Part model, mm, in its own coordinate system. Face numbers are marked on the shaded views. Round coordinates to 2 decimals unless told otherwise and drop trailing zeros. Order: outer loops, then holes, each group sorted by start corner. A loop starts at its lowest first (then second) coordinate and runs counter-clockwise, first axis right, second up. Notation, with made-up numbers: (87.5, 77) - (141.5, 77) arc R17 ccw to (141.5, 96) - close; hole circle Ø2 at (25.25, -23). An arc over 180 degrees is marked (long way). Return JSON: item names as keys, results as strings. Group by question number.
Item 1: Saw through at B-B on z = 1.35. List the corners of the cut face in (x, y).
Item 2: Saw through at C-C on y = 0.5. List the corners of the cut face in (x, z) (3 decimals), and give its area (3 significant figures).
Item 3: Probe probe 1 along Y at (x, z) = (0, 0.95); probe 2 along Z at (x, y) = (-3.75, -1); probe 3 along Z at (x, y) = (0.75, -3.75). List the from-to ranges inside material, lowest first.
Item 4: Two-plate mould, pull along Y, no slides. Class the marked faces 1, 2 and 3: released by +Y, released by -Y, zero draft, split by the parting line, or undercut.
Item 5: Saw through at A-A on x = 0. List the corners of the cut face in (y, z).
Item 6: Saw through at D-D on x = 5.25. List the corners of the cut face in (y, z), and give its area (3 significant figures).
Item 7: Drop a flat-ended pin along its axis: pin 1 (1 mm diameter, centred on y = -3, z = 1.5, fed in from -X). Give the stop position or say it passes through.
```python
from build123d import *

# Parameters (mm, degrees)
F0_R          = 2.3
F1_DEPTH      = 3
F2_R          = 72.2
F3_DEPTH      = 25
F3_DEPTH_BACK = 25


with BuildPart() as f1:
    # F0 (on Top) → F1 (new body)
    with BuildSketch(Plane.XY):
        with BuildLine():
            Line((-6.5268066341, 0), (-3.8303570799, -3.2137773166))
            ThreePointArc((-3.8303570799, -3.2137773166), (0, -5), (3.8303570799, -3.2137773166))
            Line((3.8303570799, -3.2137773166), (6.5268066341, 0))
            Line((6.5268066341, 0), (3.8303570799, 3.2137773166))
            ThreePointArc((3.8303570799, 3.2137773166), (0, 5), (-3.8303570799, 3.2137773166))
            Line((-3.8303570799, 3.2137773166), (-6.5268066341, 0))
        make_face()
        Circle(F0_R, mode=Mode.SUBTRACT)
    extrude(amount=F1_DEPTH)

    # F2 (on Front) → F3 (cut, two sides)
    with BuildSketch(Plane.XZ) as f3_sk:
        with Locations((0, 73.7)):
            Circle(F2_R)
    extrude(amount=-F3_DEPTH, mode=Mode.SUBTRACT)
    extrude(f3_sk.sketch, amount=F3_DEPTH_BACK, mode=Mode.SUBTRACT)


solid = f1.part
```
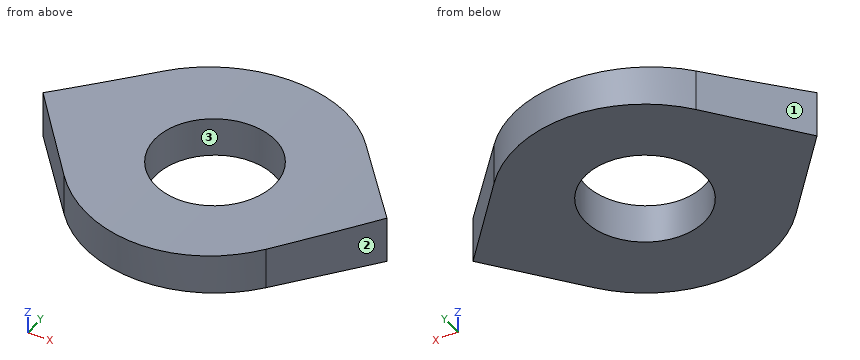
Filled in:
{
 "1": {"outline": "(-6.53, 0) - (-3.83, -3.21) arc R5 ccw to (3.83, -3.21) - (6.53, 0) - (3.83, 3.21) arc R5 ccw to (-3.83, 3.21) - close; hole circle Ø4.6 at (0, 0)"},
 "2": {"outline": "(-6.107, 0) - (-2.245, 0) - (-2.245, 1.535) arc R72.2 cw to (-6.107, 1.759) - close; (2.245, 0) - (6.107, 0) - (6.107, 1.759) arc R72.2 cw to (2.245, 1.535) - close", "area": "12.6 mm^2"},
 "3": {"probe 1": "y = -5 to -2.3, 2.3 to 5", "probe 2": "z = 0 to 1.6", "probe 3": "z = 0 to 1.5"},
 "4": {"face 1": "released by +Y", "face 2": "released by -Y", "face 3": "undercut"},
 "5": {"outline": "(-5, 0) - (-2.3, 0) - (-2.3, 1.5) - (-5, 1.5) - close; (2.3, 0) - (5, 0) - (5, 1.5) - (2.3, 1.5) - close"},
 "6": {"outline": "(-1.52, 0) - (1.52, 0) - (1.52, 1.69) - (-1.52, 1.69) - close", "area": "5.15 mm^2"},
 "7": {"pin 1": "stops at x = -4.43"}
}
